Read the model definition and answer for the solid it produces. Units are mm, in the model's axes. Face numbers are marked on the shaded views. A direction names the side the tool comes from. Coordinates: 2 decimals unless noted, no trailing zeros. Loops run counter-clockwise (first coordinate to the right, second up) from the corner with the lowest first, then second, coordinate; pieces in that order, holes last. Notation, with made-up numbers: (28, 71) - (33, 71) arc R4 ccw to (33, 77) - close; hole circle Ø5 at (45, 11). An arc over 180 degrees is marked (long way). Use one line per item in the form item = value. Start each with the question number.
1) A cutting plane is placed at A-A (y = -2). Give the vertices of the cut face in (x, z), and give its area (3 significant figures).
2) A cutting plane is placed at C-C (z = 3). Give the vertices of the cut face in (x, y), and give its area (3 significant figures).
3) A cutting plane is placed at B-B (z = 14). Give the vertices of the cut face in (x, y).
4) Which of the six approach directions +Z, -Z, +X, -X, +Y, -Y give full straight-line access (tool end or side, diameter ignored) to the marked faces 4, 5 and 6?
5) The mould has two halves that part along X. Classify the marked faces 1, 2 and 3: released by +X, released by -X, zero draft, split by the parting line, or undercut.
6) Consider line 1 (X direction, y = -22, z = 21); line 2 (X direction, y = -11.5, z = 18.5); line 3 (Z direction, x = 0.5, y = -13.75). Determine where each line is inside the solid, lowest interval first.
7) Each of these flat-tipped pins is pushed along its axis until it touches: P1, Ø12, axis at x = -13, y = -8.5, coming from the +Z side; P2, Ø4, axis at x = 13.5, z = 19.5, coming from the -Y side; P3, Ø6, axis at y = -20, z = 23, coming from the +X side; P4, Ø6, axis at x = 19, z = 13.5, coming from the -Y side. Where does it stop, or does it pass through?
8) A cutting plane is placed at D-D (x = 23). Give the vertices of the cut face in (y, z).
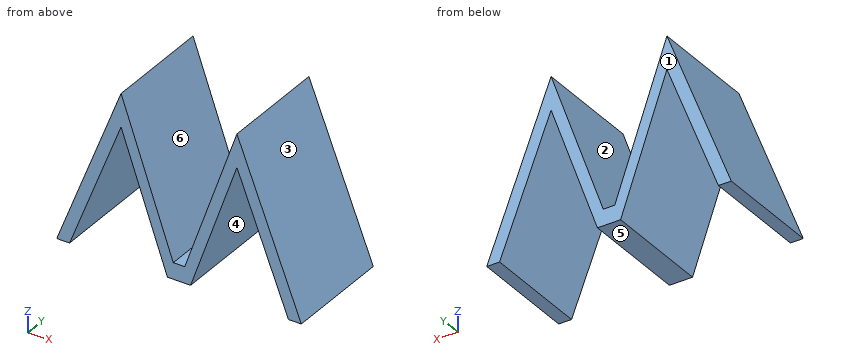
from build123d import *

# Parameters (mm, degrees)
F1_DEPTH = 25
F2_W     = 5.325386
F2_H     = 3.749341
F3_DEPTH = 25


with BuildPart() as f1:
    # F0 (on Front) → F1 (new body)
    with BuildSketch(Plane.XZ):
        Polygon((-13.309799, 37.808198), (-28.098464, 0), (-25.139917, 0), (-13.309799, 30.244477), (-2.662693, 0), (0, 0), align=None)
        Polygon((13.309799, 37.808198), (0, 0), (2.662693, 0), (13.309799, 30.244477), (25.139917, 0), (28.098464, 0), align=None)
    extrude(amount=F1_DEPTH)

    # F2 (on face) → F3 (join)
    with BuildSketch(Plane.XZ.offset(25)):
        with Locations((0, 1.87467)):
            Rectangle(F2_W, F2_H)
    extrude(amount=-F3_DEPTH)


solid = f1.part
Found:
q1.outline = (-28.1, 0) - (-25.14, 0) - (-13.31, 30.24) - (-2.66, 0) - (2.66, 0) - (13.31, 30.24) - (25.14, 0) - (28.1, 0) - (13.31, 37.81) - (1.32, 3.75) - (-1.32, 3.75) - (-13.31, 37.81) - close
q1.area = 387 mm^2
q2.outline = (-26.93, -25) - (-23.97, -25) - (-23.97, 0) - (-26.93, 0) - close; (-3.72, -25) - (3.72, -25) - (3.72, 0) - (-3.72, 0) - close; (23.97, -25) - (26.93, -25) - (26.93, 0) - (23.97, 0) - close
q2.area = 334 mm^2
q3.outline = (-22.62, -25) - (-19.66, -25) - (-19.66, 0) - (-22.62, 0) - close; (-7.59, -25) - (-4.93, -25) - (-4.93, 0) - (-7.59, 0) - close; (4.93, -25) - (7.59, -25) - (7.59, 0) - (4.93, 0) - close; (19.66, -25) - (22.62, -25) - (22.62, 0) - (19.66, 0) - close
q4.face_4 = -Z, +Y, -Y
q4.face_5 = -Z, +X, -X, +Y, -Y
q4.face_6 = +Z, +Y, -Y
q5.face_1 = zero draft
q5.face_2 = undercut
q5.face_3 = released by +X
q6.line_1 = -19.88 to -16.93, -10.06 to -7.39, 7.39 to 10.06, 16.93 to 19.88
q6.line_2 = -20.86 to -17.9, -9.18 to -6.51, 6.51 to 9.18, 17.9 to 20.86
q6.line_3 = 0 to 3.75
q7.P1 = 37.81
q7.P2 = through
q7.P3 = 20.28
q7.P4 = -25
q8.outline = (-25, 5.47) - (0, 5.47) - (0, 13.03) - (-25, 13.03) - close
